```python
from build123d import *

# Parameters (mm, degrees)
F0_R     = 4.5
F0_R_2   = 17.5
F1_DEPTH = 9
F0_R_3   = 13.5
F0_R_4   = 12.5
F2_DEPTH = 29
F3_DEPTH = 27
F4_SIZE  = 1


with BuildPart() as f1:
    # F0 (on Front) → F1 (new body)
    with BuildSketch(Plane.XZ):
        with BuildLine():
            Line((10.116541, -35.819212), (20.517576, -11.457707))
            ThreePointArc((20.517576, -11.457707), (23.5, 0), (20.517576, 11.457707))
            Line((20.517576, 11.457707), (10.116541, 35.819212))
            ThreePointArc((10.116541, 35.819212), (0, 42.5), (-10.116541, 35.819212))
            Line((-10.116541, 35.819212), (-20.517576, 11.457707))
            ThreePointArc((-20.517576, 11.457707), (-23.5, 0), (-20.517576, -11.457707))
            Line((-20.517576, -11.457707), (-10.116541, -35.819212))
            ThreePointArc((-10.116541, -35.819212), (0, -42.5), (10.116541, -35.819212))
        make_face()
        with Locations((0, -31.5)):
            Circle(F0_R, mode=Mode.SUBTRACT)
        Circle(F0_R_2, mode=Mode.SUBTRACT)
        with Locations((0, 31.5)):
            Circle(F0_R, mode=Mode.SUBTRACT)
    extrude(amount=F1_DEPTH)

    # F0 (on Front) → F2 (join)
    with BuildSketch(Plane.XZ):
        Circle(F0_R_2)
        Circle(F0_R_3, mode=Mode.SUBTRACT)
        Circle(F0_R_3)
        Circle(F0_R_4, mode=Mode.SUBTRACT)
    extrude(amount=F2_DEPTH)

    # F0 (on Front) → F3 (cut)
    with BuildSketch(Plane.XZ):
        Circle(F0_R_3)
        Circle(F0_R_4, mode=Mode.SUBTRACT)
    extrude(amount=F3_DEPTH, mode=Mode.SUBTRACT)

    # F4
    f4_edges = [f1.edges().sort_by_distance(p)[0] for p in [
        (-17.5, -29, 0),
        (23.5, -9, 0),
        (15.317059, -9, -23.63846),
        (15.317059, -9, 23.63846),
    ]]
    chamfer(f4_edges, length=F4_SIZE)


solid = f1.part
```
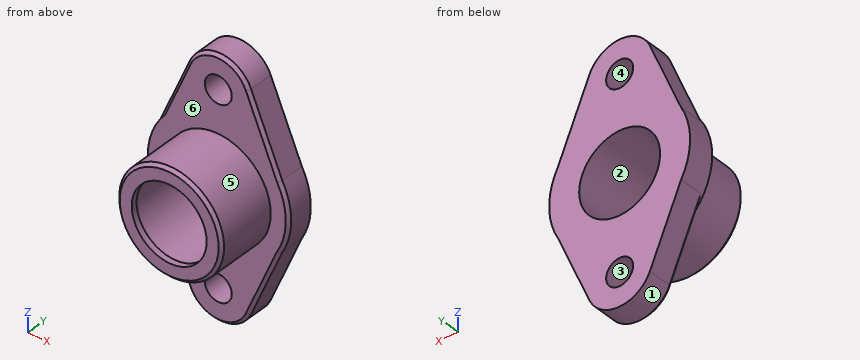
Geometry: final body of the model. Coordinates: model frame, mm. Face numbers are marked on the shaded views. A direction names the side the tool comes from. Round coordinates to 2 decimals unless told otherwise and drop trailing zeros. Order: outer loops, then holes, each group sorted by start corner. A loop starts at its lowest first (then second) coordinate and runs counter-clockwise, first axis right, second up. Notation, with made-up numbers: (32, -33) -> (54, -33) arc R18 ccw to (54, -20) -> close; hole circle Ø6 at (-24, -12). An arc over 180 degrees is marked (long way). Use one line per item in the form item = value. Start each with the question number.
1. Cut plane A-A (z = 0). Return the cut outline in (x, y), then the cut area to 4 significant figures.
2. Cut plane C-C (y = -6). Return the cut outline in (x, z), then the cut area to 3 significant figures.
3. Reachability of the marked faces 1 and 2 from +Z, -Z, +X, -X, +Y, -Y: full face, straight path, thin tool, end or side. Return the list, or none.
4. Cut plane B-B (x = 0). Return the cut outline in (y, z).
5. Cut plane D-D (y = -13). Return the cut outline in (x, z).
6. Line query: probe 1 along Z at (x, y) = (0, -14.5); probe 2 along Y at (x, z) = (-10.5, -28.5); probe 3 along Z at (x, y) = (-9, -5.25). Output: solid intervals per line, ascending.
7. Draft query along X for the marked faces 3, 4, 5 and 6. Return one class per face: pulls with the +X half, pulls with the -X half, needs draft (parallel to the pull), parting line crosses it, or undercut.
8. Pin query (flat end, axial travel): pin 1 Ø24.5 at (x, z) = (0, 0) entering from -Y; pin 2 Ø10 at (x, z) = (3.5, 26) entering from -Y; pin 3 Ø5 at (x, y) = (-12.5, -22.5) entering from +Z; pin 4 Ø10 at (x, y) = (3.5, -19.5) entering from +Z. Return the tip coordinate at first contact, or that it passes through.
Solution:
q1.outline = (-23.5, -9) -> (-17.5, -9) -> (-17.5, -28) -> (-16.5, -29) -> (-12.5, -29) -> (-12.5, -27) -> (-13.5, -27) -> (-13.5, 0) -> (-23.5, 0) -> close; (12.5, -29) -> (16.5, -29) -> (17.5, -28) -> (17.5, -9) -> (22.5, -9) -> (23.5, -8) -> (23.5, 0) -> (13.5, 0) -> (13.5, -27) -> (12.5, -27) -> close
q1.area = 342.5 mm^2
q2.outline = (-20.52, -11.46) -> (-10.12, -35.82) arc R11 ccw to (10.12, -35.82) -> (20.52, -11.46) arc R23.5 ccw to (20.52, 11.46) -> (10.12, 35.82) arc R11 ccw to (-10.12, 35.82) -> (-20.52, 11.46) arc R23.5 ccw to start; hole circle Ø27 at (0, 0); hole circle Ø9 at (0, -31.5); hole circle Ø9 at (0, 31.5)
q2.area = 2,020 mm^2
q3.face_1 = -Z, +Y, -Y
q3.face_2 = +Y
q4.outline = (-29, -16.5) -> (-28, -17.5) -> (-9, -17.5) -> (-9, -27) -> (0, -27) -> (0, -13.5) -> (-27, -13.5) -> (-27, -12.5) -> (-29, -12.5) -> close; (-29, 12.5) -> (-27, 12.5) -> (-27, 13.5) -> (0, 13.5) -> (0, 27) -> (-9, 27) -> (-9, 17.5) -> (-28, 17.5) -> (-29, 16.5) -> close; (-9, -41.5) -> (-8, -42.5) -> (0, -42.5) -> (0, -36) -> (-9, -36) -> close; (-9, 36) -> (0, 36) -> (0, 42.5) -> (-8, 42.5) -> (-9, 41.5) -> close
q5.outline = circle Ø35 at (0, 0); hole circle Ø27 at (0, 0)
q6.probe_1 = -17.5 to -13.5, 13.5 to 17.5
q6.probe_2 = -9 to 0
q6.probe_3 = -37.82 to -10.06, 10.06 to 37.82
q7.face_3 = undercut
q7.face_4 = undercut
q7.face_5 = parting line crosses it
q7.face_6 = needs draft
q8.pin_1 = through
q8.pin_2 = -9
q8.pin_3 = 14.36
q8.pin_4 = 17.5
